Verification items for the finished model (mm, model axes). A direction names the side the tool comes from. Round coordinates to 2 decimals unless told otherwise and drop trailing zeros. Order: outer loops, then holes, each group sorted by start corner. A loop starts at its lowest first (then second) coordinate and runs counter-clockwise, first axis right, second up.
```python
from build123d import *

# Parameters (mm, degrees)
BOSS_EXTRUDE1_DEPTH = 13.9954
SKETCH2_R           = 2.38125
BOSS_EXTRUDE2_DEPTH = 3.175


with BuildPart() as part:
    # Sketch1 → Boss-Extrude1 (new body, symmetric)
    with BuildSketch(Plane(origin=(0, 0, 0), x_dir=(1, 0, 0), z_dir=(0, 1, 0))):
        Polygon((1.374815329, -2.38125), (2.749630657, 0), (1.374815329, 2.38125), (-1.374815329, 2.38125), (-2.749630657, 0), (-1.374815329, -2.38125), align=None)
    extrude(amount=BOSS_EXTRUDE1_DEPTH, both=True)

    # Sketch2 → Boss-Extrude2 (add)
    with BuildSketch(Plane(origin=(0, 13.9954, 0), x_dir=(1, 0, 0), z_dir=(0, 1, 0))):
        Circle(SKETCH2_R)
    boss_extrude2 = extrude(amount=BOSS_EXTRUDE2_DEPTH)

    # Mirror1: Boss-Extrude2 across plane
    add(boss_extrude2.mirror(Plane.ZX))


solid = part.part
```
1) Sectioned sample at A-A on y = 3.5. Record the cut outline in (x, z).
2) Go/stop test with flat-tipped pins: pin 1 Ø1.5 at (y, z) = (-1, -0.5) entering from +X; pin 2 Ø1 at (y, z) = (-5, -1) entering from +X; pin 3 Ø2 at (y, z) = (-7.5, -2) entering from -X. Record where each tip stops, or that it passes through.
3) Sectioned sample at C-C on z = 1.95. Record the cut outline in (x, y), then the cut area to 3 significant figures.
4) Scan lines: probe 1 along X at (y, z) = (-6, 1.2); probe 2 along X at (y, z) = (-9.5, -0.5); probe 3 along Z at (x, y) = (-1.6, 5). Record each from-to range of solid material in increasing order.
5) Tool access check on faces 1 (the flat face through (-1.3, -13.995, 2.2)), 2 (the flat face through (1.3, 13.995, -2.2)), 3 (the flat face through (-1.3, 13.995, -2.2)), 4 (the flat face through (-1.3, 13.995, 2.2)). Record the directions out of +Z, -Z, +X, -X, +Y, -Y that give a thin tool (end or side, any length) a straight path to the whole face; none if there is none.
Returned:
1. outline: (-2.75, 0) - (-1.37, -2.38) - (1.37, -2.38) - (2.75, 0) - (1.37, 2.38) - (-1.37, 2.38) - close
2. pin 1: stops at x = 2.75
2. pin 2: stops at x = 2.46
2. pin 3: stops at x = -2.17
3. outline: (-1.62, -14) - (-1.37, -14) - (-1.37, -17.17) - (1.37, -17.17) - (1.37, -14) - (1.62, -14) - (1.62, 14) - (1.37, 14) - (1.37, 17.17) - (-1.37, 17.17) - (-1.37, 14) - (-1.62, 14) - close
3. area: 108 mm2
4. probe 1: x = -2.06 to 2.06
4. probe 2: x = -2.46 to 2.46
4. probe 3: z = -1.99 to 1.99
5. face 1: +Z, -X, -Y
5. face 2: -Z, +X, +Y
5. face 3: -Z, -X, +Y
5. face 4: +Z, -X, +Y
